Model file for the job. Use its own axes, mm. A direction names the side the tool comes from. Coordinates: 2 decimals unless noted, no trailing zeros. Loops run counter-clockwise (first coordinate to the right, second up) from the corner with the lowest first, then second, coordinate; pieces in that order, holes last.
from build123d import *

# Parameters (mm, degrees)
BOSS_EXTRUDE1_DEPTH       = 10
F_4_40_TAPPED_HOLE1_D     = 2.2606
F_4_40_TAPPED_HOLE1_DEPTH = 10
F_4_40_TAPPED_HOLE1_TIP   = 0.679152758
F_4_40_TAPPED_HOLE2_D     = 2.2606
F_4_40_TAPPED_HOLE2_DEPTH = 10
F_4_40_TAPPED_HOLE2_TIP   = 0.679152758
F_4_40_TAPPED_HOLE3_D     = 2.2606
F_4_40_TAPPED_HOLE3_DEPTH = 10
F_4_40_TAPPED_HOLE3_TIP   = 0.679152758


with BuildPart() as part:
    # Sketch1 → Boss-Extrude1 (new body)
    with BuildSketch(Plane(origin=(0, 0, 0), x_dir=(1, 0, 0), z_dir=(0, 1, 0))):
        Polygon((0, 0), (0, 25), (25, 25), (25, 15), (10, 0), align=None)
    extrude(amount=BOSS_EXTRUDE1_DEPTH)

    # #4-40 Tapped Hole1
    with Locations(Plane.ZY):
        with Locations((-15, 5)):
            Hole(F_4_40_TAPPED_HOLE1_D / 2, depth=F_4_40_TAPPED_HOLE1_DEPTH)
            with Locations((0, 0, -(F_4_40_TAPPED_HOLE1_DEPTH + F_4_40_TAPPED_HOLE1_TIP / 2))):  # 118° drill point
                Cone(0, F_4_40_TAPPED_HOLE1_D / 2, F_4_40_TAPPED_HOLE1_TIP, mode=Mode.SUBTRACT)

    # #4-40 Tapped Hole2
    with Locations(Plane(origin=(0, 10, 0), x_dir=(1, 0, 0), z_dir=(0, 1, 0))):
        with Locations((13, 20)):
            Hole(F_4_40_TAPPED_HOLE2_D / 2, depth=F_4_40_TAPPED_HOLE2_DEPTH)
            with Locations((0, 0, -(F_4_40_TAPPED_HOLE2_DEPTH + F_4_40_TAPPED_HOLE2_TIP / 2))):  # 118° drill point
                Cone(0, F_4_40_TAPPED_HOLE2_D / 2, F_4_40_TAPPED_HOLE2_TIP, mode=Mode.SUBTRACT)

    # #4-40 Tapped Hole3
    with Locations(Plane(origin=(0, 0, -25), x_dir=(-1, 0, 0), z_dir=(0, 0, -1))):
        with Locations((-18, 5)):
            Hole(F_4_40_TAPPED_HOLE3_D / 2, depth=F_4_40_TAPPED_HOLE3_DEPTH)
            with Locations((0, 0, -(F_4_40_TAPPED_HOLE3_DEPTH + F_4_40_TAPPED_HOLE3_TIP / 2))):  # 118° drill point
                Cone(0, F_4_40_TAPPED_HOLE3_D / 2, F_4_40_TAPPED_HOLE3_TIP, mode=Mode.SUBTRACT)


solid = part.part
Q1. Flat gauge pin, fed straight in: P1, Ø1.4, axis at x = 18, y = 5, coming from the +Z side. Where does the tip first touch, or does it go through?
Answers:
P1: stops at z = -7.3
Q2. Slice it at D-D (y = 7.5). List the corners of the cut face in (x, z), and give its area (3 significant figures).
Answers:
outline: (0, -25) - (25, -25) - (25, -15) - (10, 0) - (0, 0) - close; hole circle Ø2.26 at (13, -20)
area: 508 mm2
Q3. Slice it at C-C (x = 3.25). List the corners of the cut face in (y, z), and give its area (3 significant figures).
Answers:
outline: (0, -25) - (10, -25) - (10, 0) - (0, 0) - close; hole circle Ø2.26 at (5, -15)
area: 246 mm2
Q4. Slice it at B-B (z = -17.5). List the corners of the cut face in (x, y).
Answers:
outline: (0, 0) - (25, 0) - (25, 10) - (0, 10) - close; hole circle Ø2.26 at (18, 5)
Q5. Mould opens along Y. For faces 4 (the flat face through (10, 0, -15)), 5 (the cylindrical face through (13.897, 4.93, -19.312)), 6 (the conical face through (18.043, 4.808, -14.439)) say: +Y half, -Y half, draft (parallel to the pull), parting line (faces both ways), or undercut.
Answers:
face 4: -Y half
face 5: draft
face 6: undercut
Q6. Slice it at A-A (z = -20). List the corners of the cut face in (x, y), and give its area (3 significant figures).
Answers:
outline: (0, 0) - (11.87, 0) - (11.87, 10) - (0, 10) - close; (14.13, 0) - (25, 0) - (25, 10) - (14.13, 10) - close; hole circle Ø2.26 at (18, 5)
area: 223 mm2
Q7. Which spindle directions (+Z, -Z, +X, -X, +Y, -Y) get a long thin tool onto all of the face, cutting with end or side? Do faces 1 (the cylindrical face through (5.07, 4.312, -14.103)), 2 (the cylindrical face through (18.522, 3.997, -19.93)), 3 (the flat face through (18, 5, -8)). Say none if no direction does.
Answers:
face 1: -X
face 2: -Z
face 3: +Z, +X, +Y, -Y
Q8. Drill centre lines: line 1 (Y direction, x = 5.25, z = -15); line 2 (X direction, y = 5, z = -19); line 3 (Z direction, x = 3.75, y = 5). Where is each one in solid material? Low to high.
Answers:
line 1: y = 0 to 3.87, 6.13 to 10
line 2: x = 0 to 12.47, 13.53 to 16.87, 19.13 to 25
line 3: z = -25 to -16.13, -13.87 to 0
